from build123d import *

# Parameters (mm, degrees)
F1_DEPTH = 63.5
F0_W     = 25.4
F0_H     = 19.05
F2_DEPTH = 25.4
F3_DEPTH = 7.9375
F5_R     = 6.35
F6_R     = 12.7
F7_DEPTH = 76.201


with BuildPart() as f1:
    # F0 (on Front) → F1 (new body, symmetric)
    with BuildSketch(Plane.XZ):
        Polygon((41.275, -9.525), (41.275, 9.525), (22.225, 9.525), (-41.275, 9.525), (-41.275, -9.525), align=None)
    extrude(amount=F1_DEPTH, both=True)

    # F0 (on Front) → F2 (join, symmetric)
    with BuildSketch(Plane.XZ):
        with BuildLine():
            Line((22.225, 9.525), (41.275, 9.525))
            Line((41.275, 9.525), (41.275, 27.0002))
            ThreePointArc((41.275, 27.0002), (45.92468, 38.22552), (57.15, 42.8752))
            Line((57.15, 42.8752), (60.325, 42.8752))
            Line((60.325, 42.8752), (60.325, 61.9252))
            Line((60.325, 61.9252), (57.15, 61.9252))
            ThreePointArc((57.15, 61.9252), (32.454296, 51.695904), (22.225, 27.0002))
            Line((22.225, 27.0002), (22.225, 9.525))
        make_face()
        with Locations((73.025, 52.4002)):
            Rectangle(F0_W, F0_H)
    extrude(amount=F2_DEPTH, both=True)

    # F0 (on Front) → F3 (join, symmetric)
    with BuildSketch(Plane.XZ):
        with BuildLine():
            Line((-41.275, 9.525), (22.225, 9.525))
            Line((22.225, 9.525), (22.225, 27.0002))
            ThreePointArc((22.225, 27.0002), (32.454296, 51.695904), (57.15, 61.9252))
            add(Edge.make_bspline(
                [(-41.275, 9.525), (-29.649258, 28.44544), (-12.466568, 62.335622), (57.15, 61.9252)],
                knots=[0, 0, 0, 0, 111.504536, 111.504536, 111.504536, 111.504536], degree=3))
        make_face()
    extrude(amount=F3_DEPTH, both=True)

    # F0 (on Front) → F4 (revolve)
    with BuildSketch(Plane.XZ):
        Polygon((85.725, 61.9252), (85.725, 42.8752), (85.725, 38.1), (111.125, 38.1), (111.125, 66.675), (85.725, 66.675), align=None)
    revolve(axis=Axis((85.725, 0, 52.4002), (0, 0, -1)))

    # F5
    f5_edges = [f1.edges().sort_by_distance(p)[0] for p in [
        (41.275, -63.5, 0),
        (-41.275, -63.5, 0),
        (-41.275, 63.5, 0),
        (41.275, 63.5, 0),
    ]]
    fillet(f5_edges, radius=F5_R)

    # F6 (on face) → F7 (cut, through all)
    with BuildSketch(Plane.XY.offset(66.675)):
        with Locations((85.725, 0)):
            Circle(F6_R)
    extrude(amount=-F7_DEPTH, mode=Mode.SUBTRACT)


solid = f1.part
Can you work these out from the model? Positions are in its coordinate system, mm. A direction names the side the tool comes from. Coordinates: 2 decimals unless noted, no trailing zeros. Order: outer loops, then holes, each group sorted by start corner. A loop starts at its lowest first (then second) coordinate and runs counter-clockwise, first axis right, second up. Notation, with made-up numbers: (53.5, -15) -> (67.5, -15) arc R23 cw to (67.5, 20) -> close; hole circle Ø5 at (13.25, -35.5). An arc over 180 degrees is marked (long way). Use one line per item in the form item = value.
Q1. Imagine slicing it at C-C, the plane y = 53.5. List the corners of the cut face in (x, z) for me (3 decimals).
From the geometry:
outline = (-41.275, -9.525) -> (41.275, -9.525) -> (41.275, 9.525) -> (-41.275, 9.525) -> close
Q2. We'd pull the mould along X, two halves only. Please class faces 4 (the face through (39.464, -61.59, 0.133)), 5 (the face through (45.8, -0.4, 38.1)), 6 (the face through (-41.275, -1, 0)): released by +X, released by -X, zero draft, split by the parting line, or undercut.
From the geometry:
face_4 = released by +X
face_5 = undercut
face_6 = released by -X
Q3. I need wall thicknesses on L1, parallel to Z at x = -2, y = -26.5 (3 decimals); L2, parallel to Z at x = 72, y = 1.5 (3 decimals); L3, parallel to Y at x = 30.5, z = 40.5. Which ranges of each line are inside material? Lowest first, please.
From the geometry:
L1 = -9.525 to 9.525
L2 = 38.1 to 66.675
L3 = -25.4 to 25.4
Q4. Imagine slicing it at A-A, the plane x = 75. List the corners of the cut face in (y, z) for me (3 decimals), then the cut area to 3 significant figures.
From the geometry:
outline = (-25.4, 42.875) -> (-23.025, 42.875) -> (-23.025, 38.1) -> (-6.802, 38.1) -> (-6.802, 66.675) -> (-23.025, 66.675) -> (-23.025, 61.925) -> (-25.4, 61.925) -> close; (6.802, 38.1) -> (23.025, 38.1) -> (23.025, 42.875) -> (25.4, 42.875) -> (25.4, 61.925) -> (23.025, 61.925) -> (23.025, 66.675) -> (6.802, 66.675) -> close
area = 1,020 mm²
Q5. Imagine slicing it at B-B, the plane y = 17. List the corners of the cut face in (x, z) for me (3 decimals), then the cut area to 3 significant figures.
From the geometry:
outline = (-41.275, -9.525) -> (41.275, -9.525) -> (41.275, 27) arc R15.875 cw to (57.15, 42.875) -> (66.853, 42.875) -> (66.853, 38.1) -> (104.597, 38.1) -> (104.597, 66.675) -> (66.853, 66.675) -> (66.853, 61.925) -> (57.15, 61.925) arc R34.925 ccw to (22.225, 27) -> (22.225, 9.525) -> (-41.275, 9.525) -> close
area = 3,930 mm²
Q6. Will these pins go through, and if not, where does the flat tip stop? P1, Ø4, axis at y = -24, z = 39, coming from the -X side; P2, Ø3, axis at x = 66, z = 51.5, coming from the +Y side; P3, Ø5, axis at y = -3.5, z = 36.5, coming from the -X side.
From the geometry:
P1 = 23.69
P2 = 25.4
P3 = -23.88
Q7. Which directions (+Z, -Z, +X, -X, +Y, -Y) give clear straight access to the entire face, cutting with the end or side of a thin tool? Please do faces 1 (the face through (22.225, 17, 18)), 2 (the face through (80, -12, 38.1)), 3 (the face through (60, -2, 61.925)).
From the geometry:
face_1 = +Z, -X, +Y
face_2 = -Z, +X, +Y, -Y
face_3 = +Z, -X
